Can you work these out from the model? Positions are in its coordinate system, mm. Face numbers are marked on the shaded views. Coordinates: 2 decimals unless noted, no trailing zeros. Write each loop counter-clockwise with the first axis right and the second up, starting at its lowest first coordinate (ties: lowest second). Pieces come first, ordered by that corner, then holes. Notation, with made-up numbers: M 38.25,75 L 85.25,75 A22 ccw 85.25,86 Z; hole C -26,11 d8. An arc over 180 degrees is marked long. Answer as a JSON object with one key per item and string values. Group by question number.
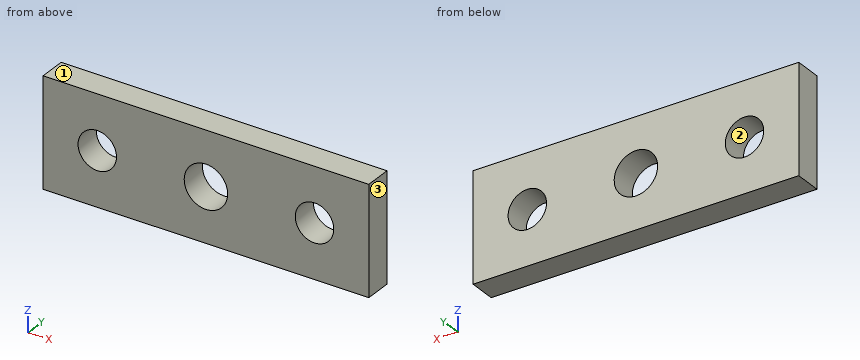
from build123d import *

# Parameters (mm, degrees)
SKETCH1_W             = 38.1
SKETCH1_H             = 12.7
BOSS_EXTRUDE1_DEPTH   = 3.175
SKETCH2_R             = 2.54
CUT_EXTRUDE1_DEPTH    = 21.329919454
F_8_CLEARANCE_HOLE1_D = 4.4958


with BuildPart() as part:
    # Sketch1 → Boss-Extrude1 (new body)
    with BuildSketch(Plane(origin=(0, 0, 0), x_dir=(1, 0, 0), z_dir=(0, 1, 0))):
        Rectangle(SKETCH1_W, SKETCH1_H)
    extrude(amount=BOSS_EXTRUDE1_DEPTH)

    # Sketch2 → Cut-Extrude1 (cut, through all)
    with BuildSketch(Plane(origin=(0, 3.175, 0), x_dir=(1, 0, 0), z_dir=(0, 1, 0))):
        with Locations(Location((0, 0, 0), (0, 0, 270))):
            Circle(SKETCH2_R)
    extrude(amount=-CUT_EXTRUDE1_DEPTH, mode=Mode.SUBTRACT)

    # #8 Clearance Hole1 (through all)
    with Locations(Plane(origin=(0, 3.175, 0), x_dir=(1, 0, 0), z_dir=(0, 1, 0))):
        with Locations((-12.7, 0), (12.7, 0)):
            Hole(F_8_CLEARANCE_HOLE1_D / 2)


solid = part.part
Q1. If we section it at A-A on z = 0: List the corners of the cut face in (x, y) for me (3 decimals).
Q2. If we section it at C-C on x = 0: List the corners of the cut face in (y, z) for me (3 decimals).
Q3. We'd pull the mould along Z, two halves only. Please class the marked faces 1, 2 and 3: pulls with the +Z half, pulls with the -Z half, needs draft (parallel to the pull), parting line crosses it, or undercut.
Q4. If we section it at B-B on y = 1.45: List the corners of the cut face in (x, z) for me, and give its area (3 significant figures).
Q5. If we section it at D-D on x = 12.7: List the corners of the cut face in (y, z) for me (3 decimals), and give its area (3 significant figures).
Q6. Please list where these lines run through material, in increasing order: L1, parallel to Z at x = -12.7, y = 2.2; L2, parallel to X at y = 0.4, z = -2; L3, parallel to X at y = 2.3, z = 1.25.
Reply:
{
 "1": {"outline": "M -19.05,0 L -14.948,0 L -14.948,3.175 L -19.05,3.175 Z; M -10.452,0 L -2.54,0 L -2.54,3.175 L -10.452,3.175 Z; M 2.54,0 L 10.452,0 L 10.452,3.175 L 2.54,3.175 Z; M 14.948,0 L 19.05,0 L 19.05,3.175 L 14.948,3.175 Z"},
 "2": {"outline": "M 0,-6.35 L 3.175,-6.35 L 3.175,-2.54 L 0,-2.54 Z; M 0,2.54 L 3.175,2.54 L 3.175,6.35 L 0,6.35 Z"},
 "3": {"face 1": "pulls with the +Z half", "face 2": "undercut", "face 3": "needs draft"},
 "4": {"outline": "M -19.05,-6.35 L 19.05,-6.35 L 19.05,6.35 L -19.05,6.35 Z; hole C -12.7,0 d4.5; hole C 0,0 d5.08; hole C 12.7,0 d4.5", "area": "432 mm^2"},
 "5": {"outline": "M 0,-6.35 L 3.175,-6.35 L 3.175,-2.248 L 0,-2.248 Z; M 0,2.248 L 3.175,2.248 L 3.175,6.35 L 0,6.35 Z", "area": "26.0 mm^2"},
 "6": {"L1": "-6.35 to -2.25, 2.25 to 6.35", "L2": "-19.05 to -13.73, -11.67 to -1.57, 1.57 to 11.67, 13.73 to 19.05", "L3": "-19.05 to -14.57, -10.83 to -2.21, 2.21 to 10.83, 14.57 to 19.05"}
}
